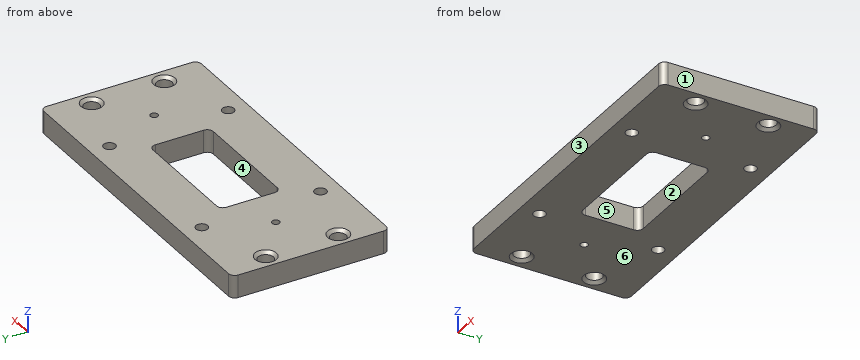
from build123d import *

# Parameters (mm, degrees)
SKETCH1_W           = 137.16
SKETCH1_H           = 66.04
BOSS_EXTRUDE1_DEPTH = 9.525
SKETCH3_R           = 2.4765
CUT_EXTRUDE1_DEPTH  = 10.525
CUT_EXTRUDE2_REACH  = 11.525
SKETCH4_R           = 3.2385
CUT_EXTRUDE3_REACH  = 11.525
SKETCH5_R           = 1.6
CUT_EXTRUDE4_REACH  = 11.525
SKETCH6_W           = 50.8
SKETCH6_H           = 25.4
FILLET1_R           = 2.54
FILLET2_R           = 2.54
CHAMFER1_SIZE       = 1.27


with BuildPart() as part:
    # Sketch1 → Boss-Extrude1 (new body)
    with BuildSketch(Plane.XY):
        Rectangle(SKETCH1_W, SKETCH1_H)
    extrude(amount=BOSS_EXTRUDE1_DEPTH)

    # Sketch3 → Cut-Extrude1 (cut, through all)
    with BuildSketch(Plane.XY.offset(9.525)):
        with Locations((-33.02, 24.892)):
            Circle(SKETCH3_R)
        with Locations((33.02, 24.892)):
            Circle(SKETCH3_R)
        with Locations((33.02, -24.892)):
            Circle(SKETCH3_R)
        with Locations((-33.02, -24.892)):
            Circle(SKETCH3_R)
    extrude(amount=-CUT_EXTRUDE1_DEPTH, mode=Mode.SUBTRACT)

    # Sketch4 → Cut-Extrude2 (cut, up to next)
    with BuildSketch(Plane.XY.offset(9.525), mode=Mode.PRIVATE) as cut_extrude2_sk1:
        with Locations((-62.23, 15.24)):
            Circle(SKETCH4_R)
    cut_extrude2_tool1 = extrude(cut_extrude2_sk1.sketch, amount=-CUT_EXTRUDE2_REACH, mode=Mode.PRIVATE) & part.part
    add(cut_extrude2_tool1.solids().sort_by_distance((-62.23, 15.24, 9.525))[0], mode=Mode.SUBTRACT)
    # Sketch4 → Cut-Extrude2 (cut, up to next)
    with BuildSketch(Plane.XY.offset(9.525), mode=Mode.PRIVATE) as cut_extrude2_sk2:
        with Locations((62.23, 15.24)):
            Circle(SKETCH4_R)
    cut_extrude2_tool2 = extrude(cut_extrude2_sk2.sketch, amount=-CUT_EXTRUDE2_REACH, mode=Mode.PRIVATE) & part.part
    add(cut_extrude2_tool2.solids().sort_by_distance((62.23, 15.24, 9.525))[0], mode=Mode.SUBTRACT)
    # Sketch4 → Cut-Extrude2 (cut, up to next)
    with BuildSketch(Plane.XY.offset(9.525), mode=Mode.PRIVATE) as cut_extrude2_sk3:
        with Locations((62.23, -15.24)):
            Circle(SKETCH4_R)
    cut_extrude2_tool3 = extrude(cut_extrude2_sk3.sketch, amount=-CUT_EXTRUDE2_REACH, mode=Mode.PRIVATE) & part.part
    add(cut_extrude2_tool3.solids().sort_by_distance((62.23, -15.24, 9.525))[0], mode=Mode.SUBTRACT)
    # Sketch4 → Cut-Extrude2 (cut, up to next)
    with BuildSketch(Plane.XY.offset(9.525), mode=Mode.PRIVATE) as cut_extrude2_sk4:
        with Locations((-62.23, -15.24)):
            Circle(SKETCH4_R)
    cut_extrude2_tool4 = extrude(cut_extrude2_sk4.sketch, amount=-CUT_EXTRUDE2_REACH, mode=Mode.PRIVATE) & part.part
    add(cut_extrude2_tool4.solids().sort_by_distance((-62.23, -15.24, 9.525))[0], mode=Mode.SUBTRACT)

    # Sketch5 → Cut-Extrude3 (cut, up to next)
    with BuildSketch(Plane.XY.offset(9.525), mode=Mode.PRIVATE) as cut_extrude3_sk1:
        with Locations((-43.5, 0)):
            Circle(SKETCH5_R)
    cut_extrude3_tool1 = extrude(cut_extrude3_sk1.sketch, amount=-CUT_EXTRUDE3_REACH, mode=Mode.PRIVATE) & part.part
    add(cut_extrude3_tool1.solids().sort_by_distance((-43.5, 0, 9.525))[0], mode=Mode.SUBTRACT)
    # Sketch5 → Cut-Extrude3 (cut, up to next)
    with BuildSketch(Plane.XY.offset(9.525), mode=Mode.PRIVATE) as cut_extrude3_sk2:
        with Locations((43.5, 0)):
            Circle(SKETCH5_R)
    cut_extrude3_tool2 = extrude(cut_extrude3_sk2.sketch, amount=-CUT_EXTRUDE3_REACH, mode=Mode.PRIVATE) & part.part
    add(cut_extrude3_tool2.solids().sort_by_distance((43.5, 0, 9.525))[0], mode=Mode.SUBTRACT)

    # Sketch6 → Cut-Extrude4 (cut, up to next)
    with BuildSketch(Plane.XY.offset(9.525), mode=Mode.PRIVATE) as cut_extrude4_sk1:
        Rectangle(SKETCH6_W, SKETCH6_H)
    cut_extrude4_tool1 = extrude(cut_extrude4_sk1.sketch, amount=-CUT_EXTRUDE4_REACH, mode=Mode.PRIVATE) & part.part
    add(cut_extrude4_tool1.solids().sort_by_distance((0, 0, 9.525))[0], mode=Mode.SUBTRACT)

    # Fillet1
    fillet1_edges = [part.edges().sort_by_distance(p)[0] for p in [
        (68.58, -33.02, 4.7625),
        (-68.58, -33.02, 4.7625),
        (-68.58, 33.02, 4.7625),
        (68.58, 33.02, 4.7625),
    ]]
    fillet(fillet1_edges, radius=FILLET1_R)

    # Fillet2
    fillet2_edges = [part.edges().sort_by_distance(p)[0] for p in [
        (25.4, 12.7, 4.7625),
        (25.4, -12.7, 4.7625),
        (-25.4, -12.7, 4.7625),
        (-25.4, 12.7, 4.7625),
    ]]
    fillet(fillet2_edges, radius=FILLET2_R)

    # Chamfer1
    chamfer1_edges = [part.edges().sort_by_distance(p)[0] for p in [
        (-65.4685, 15.24, 0),
        (-65.4685, 15.24, 9.525),
        (58.9915, 15.24, 0),
        (58.9915, 15.24, 9.525),
        (58.9915, -15.24, 0),
        (58.9915, -15.24, 9.525),
        (-65.4685, -15.24, 0),
        (-65.4685, -15.24, 9.525),
    ]]
    chamfer(chamfer1_edges, length=CHAMFER1_SIZE)


solid = part.part
Could you check a few things on this model? Use its own coordinates, in mm. Face numbers are marked on the shaded views. A direction names the side the tool comes from. Give positions to 0.01 mm unless a question says otherwise; leave off trailing zeros. Loops run counter-clockwise (first coordinate to the right, second up) from the corner with the lowest first, then second, coordinate; pieces in that order, holes last. Notation, with made-up numbers: (40.25, 20) -> (65.25, 20) arc R18 ccw to (65.25, 49) -> close; hole circle Ø11 at (60.25, 4). An arc over 180 degrees is marked (long way). Return JSON: item names as keys, results as strings.
Item 1: Which directions (+Z, -Z, +X, -X, +Y, -Y) give clear straight access to the entire face, cutting with the end or side of a thin tool? Please do the marked faces 5 and 6.
Geometry results:
{"face 5": "+Z, -Z", "face 6": "-Z, +X, -X, +Y, -Y"}
Item 2: If we section it at D-D on x = -43.5: List the corners of the cut face in (y, z) for me (3 decimals), plus the area to 3 significant figures.
Geometry results:
{"outline": "(-33.02, 0) -> (-1.6, 0) -> (-1.6, 9.525) -> (-33.02, 9.525) -> close; (1.6, 0) -> (33.02, 0) -> (33.02, 9.525) -> (1.6, 9.525) -> close", "area": "599 mm²"}
Item 3: We'd pull the mould along X, two halves only. Please class the marked faces 1, 2, 3 and 4: +X half, -X half, draft (parallel to the pull), parting line (faces both ways), or undercut.
Geometry results:
{"face 1": "+X half", "face 2": "undercut", "face 3": "draft", "face 4": "undercut"}
Item 4: If we section it at B-B on y = 0: List the corners of the cut face in (x, z) for me (3 decimals), plus the area to 3 significant figures.
Geometry results:
{"outline": "(-68.58, 0) -> (-45.1, 0) -> (-45.1, 9.525) -> (-68.58, 9.525) -> close; (-41.9, 0) -> (-25.4, 0) -> (-25.4, 9.525) -> (-41.9, 9.525) -> close; (25.4, 0) -> (41.9, 0) -> (41.9, 9.525) -> (25.4, 9.525) -> close; (45.1, 0) -> (68.58, 0) -> (68.58, 9.525) -> (45.1, 9.525) -> close", "area": "762 mm²"}
Item 5: If we section it at A-A on x = -11: List the corners of the cut face in (y, z) for me (3 decimals), plus the area to 3 significant figures.
Geometry results:
{"outline": "(-33.02, 0) -> (-12.7, 0) -> (-12.7, 9.525) -> (-33.02, 9.525) -> close; (12.7, 0) -> (33.02, 0) -> (33.02, 9.525) -> (12.7, 9.525) -> close", "area": "387 mm²"}
Item 6: I need wall thicknesses on L1, parallel to Y at x = -33.02, z = 7.5; L2, parallel to X at y = 25, z = 9; L3, parallel to Y at x = -62.23, z = 6.5. Which ranges of each line are inside material? Lowest first, please. Write a range as from..to.
Geometry results:
{"L1": "y = -33.02..-27.37, -22.42..22.42, 27.37..33.02", "L2": "x = -68.58..-35.49, -30.55..30.55, 35.49..68.58", "L3": "y = -33.02..-18.48, -12..12, 18.48..33.02"}
Item 7: I'm going to push flat-ended pins straight in: pin 1 (8.5 mm diameter, centred on x = -62.23, y = 15.24, fed in from +Z); pin 2 (8.5 mm diameter, centred on x = 62.23, y = -15.24, fed in from -Z). Where does each tip first touch, or does it pass through?
Geometry results:
{"pin 1": "stops at z = 9.27", "pin 2": "stops at z = 0.26"}
Item 8: If we section it at C-C on x = 62.23: List the corners of the cut face in (y, z) for me (1 decimal).
Geometry results:
{"outline": "(-33, 0) -> (-19.7, 0) -> (-18.5, 1.3) -> (-18.5, 8.3) -> (-19.7, 9.5) -> (-33, 9.5) -> close; (-12, 1.3) -> (-10.7, 0) -> (10.7, 0) -> (12, 1.3) -> (12, 8.3) -> (10.7, 9.5) -> (-10.7, 9.5) -> (-12, 8.3) -> close; (18.5, 1.3) -> (19.7, 0) -> (33, 0) -> (33, 9.5) -> (19.7, 9.5) -> (18.5, 8.3) -> close"}
